from build123d import *

# Parameters (mm, degrees)
F0_R      = 3
F0_R_2    = 0.508
F0_R_3    = 1.375
F3_DEPTH  = 1.2
F4_DEPTH  = 1
F1_W      = 3
F1_H      = 16
F5_DEPTH  = 1
F1_W_2    = 8
F1_H_2    = 5.5
F6_DEPTH  = 2.5
F1_W_3    = 11
F1_H_3    = 7.5
F7_DEPTH  = 3
F8_DEPTH  = 1.2
F1_W_4    = 1.2
F1_H_4    = 8.5
F9_DEPTH  = 1
F2_W      = 12
F2_H      = 12
F2_W_2    = 2.032
F2_H_2    = 1.27
F2_W_3    = 1.27
F2_H_3    = 2.032
F2_W_4    = 2
F2_H_4    = 3
F2_W_5    = 5
F2_W_6    = 3
F2_H_5    = 2.5
F2_W_7    = 2.5
F2_H_6    = 2
F2_W_8    = 1.524
F2_H_7    = 3.048
F10_DEPTH = 1


with BuildPart() as f3:
    # F0 (on Top) → F3 (new body)
    with BuildSketch(Plane.XY):
        with BuildLine():
            ThreePointArc((32.5, 12), (31.62132, 14.12132), (29.5, 15))
            Line((29.5, 15), (-29.5, 15))
            ThreePointArc((-29.5, 15), (-31.62132, 14.12132), (-32.5, 12))
            Line((-32.5, 12), (-32.5, -12))
            ThreePointArc((-32.5, -12), (-31.62132, -14.12132), (-29.5, -15))
            Line((-29.5, -15), (29.5, -15))
            ThreePointArc((29.5, -15), (31.62132, -14.12132), (32.5, -12))
            Line((32.5, -12), (32.5, 12))
        make_face()
        with Locations((-29, -11.5)):
            Circle(F0_R, mode=Mode.SUBTRACT)
        with Locations((29, -11.5)):
            Circle(F0_R, mode=Mode.SUBTRACT)
        with Locations((-24.13, 10.23)):
            Circle(F0_R_2, mode=Mode.SUBTRACT)
        with Locations((-21.59, 10.23)):
            Circle(F0_R_2, mode=Mode.SUBTRACT)
        with Locations((-19.05, 10.23)):
            Circle(F0_R_2, mode=Mode.SUBTRACT)
        with Locations((-16.51, 10.23)):
            Circle(F0_R_2, mode=Mode.SUBTRACT)
        with Locations((-29, 11.5)):
            Circle(F0_R, mode=Mode.SUBTRACT)
        with Locations((-24.13, 12.77)):
            Circle(F0_R_2, mode=Mode.SUBTRACT)
        with Locations((-21.59, 12.77)):
            Circle(F0_R_2, mode=Mode.SUBTRACT)
        with Locations((-19.05, 12.77)):
            Circle(F0_R_2, mode=Mode.SUBTRACT)
        with Locations((-16.51, 12.77)):
            Circle(F0_R_2, mode=Mode.SUBTRACT)
        with Locations((-13.97, 10.23)):
            Circle(F0_R_2, mode=Mode.SUBTRACT)
        with Locations((-11.43, 10.23)):
            Circle(F0_R_2, mode=Mode.SUBTRACT)
        with Locations((-8.89, 10.23)):
            Circle(F0_R_2, mode=Mode.SUBTRACT)
        with Locations((-6.35, 10.23)):
            Circle(F0_R_2, mode=Mode.SUBTRACT)
        with Locations((-3.81, 10.23)):
            Circle(F0_R_2, mode=Mode.SUBTRACT)
        with Locations((-1.27, 10.23)):
            Circle(F0_R_2, mode=Mode.SUBTRACT)
        with Locations((-13.97, 12.77)):
            Circle(F0_R_2, mode=Mode.SUBTRACT)
        with Locations((-11.43, 12.77)):
            Circle(F0_R_2, mode=Mode.SUBTRACT)
        with Locations((-8.89, 12.77)):
            Circle(F0_R_2, mode=Mode.SUBTRACT)
        with Locations((-6.35, 12.77)):
            Circle(F0_R_2, mode=Mode.SUBTRACT)
        with Locations((-3.81, 12.77)):
            Circle(F0_R_2, mode=Mode.SUBTRACT)
        with Locations((-1.27, 12.77)):
            Circle(F0_R_2, mode=Mode.SUBTRACT)
        with Locations((21.59, 5.15)):
            Circle(F0_R_2, mode=Mode.SUBTRACT)
        with Locations((24.13, 5.15)):
            Circle(F0_R_2, mode=Mode.SUBTRACT)
        with Locations((1.27, 10.23)):
            Circle(F0_R_2, mode=Mode.SUBTRACT)
        with Locations((3.81, 10.23)):
            Circle(F0_R_2, mode=Mode.SUBTRACT)
        with Locations((6.35, 10.23)):
            Circle(F0_R_2, mode=Mode.SUBTRACT)
        with Locations((8.89, 10.23)):
            Circle(F0_R_2, mode=Mode.SUBTRACT)
        with Locations((11.43, 10.23)):
            Circle(F0_R_2, mode=Mode.SUBTRACT)
        with Locations((13.97, 10.23)):
            Circle(F0_R_2, mode=Mode.SUBTRACT)
        with Locations((1.27, 12.77)):
            Circle(F0_R_2, mode=Mode.SUBTRACT)
        with Locations((3.81, 12.77)):
            Circle(F0_R_2, mode=Mode.SUBTRACT)
        with Locations((6.35, 12.77)):
            Circle(F0_R_2, mode=Mode.SUBTRACT)
        with Locations((8.89, 12.77)):
            Circle(F0_R_2, mode=Mode.SUBTRACT)
        with Locations((11.43, 12.77)):
            Circle(F0_R_2, mode=Mode.SUBTRACT)
        with Locations((13.97, 12.77)):
            Circle(F0_R_2, mode=Mode.SUBTRACT)
        with Locations((21.59, 7.69)):
            Circle(F0_R_2, mode=Mode.SUBTRACT)
        with Locations((24.13, 7.69)):
            Circle(F0_R_2, mode=Mode.SUBTRACT)
        with Locations((16.51, 10.23)):
            Circle(F0_R_2, mode=Mode.SUBTRACT)
        with Locations((19.05, 10.23)):
            Circle(F0_R_2, mode=Mode.SUBTRACT)
        with Locations((21.59, 10.23)):
            Circle(F0_R_2, mode=Mode.SUBTRACT)
        with Locations((24.13, 10.23)):
            Circle(F0_R_2, mode=Mode.SUBTRACT)
        with Locations((16.51, 12.77)):
            Circle(F0_R_2, mode=Mode.SUBTRACT)
        with Locations((19.05, 12.77)):
            Circle(F0_R_2, mode=Mode.SUBTRACT)
        with Locations((21.59, 12.77)):
            Circle(F0_R_2, mode=Mode.SUBTRACT)
        with Locations((24.13, 12.77)):
            Circle(F0_R_2, mode=Mode.SUBTRACT)
        with Locations((29, 11.5)):
            Circle(F0_R, mode=Mode.SUBTRACT)
        with Locations((-29, -11.5)):
            Circle(F0_R)
        with Locations((-29, -11.5)):
            Circle(F0_R_3, mode=Mode.SUBTRACT)
        with Locations((-29, 11.5)):
            Circle(F0_R)
        with Locations((-29, 11.5)):
            Circle(F0_R_3, mode=Mode.SUBTRACT)
        with Locations((29, 11.5)):
            Circle(F0_R)
        with Locations((29, 11.5)):
            Circle(F0_R_3, mode=Mode.SUBTRACT)
        with Locations((29, -11.5)):
            Circle(F0_R)
        with Locations((29, -11.5)):
            Circle(F0_R_3, mode=Mode.SUBTRACT)
    extrude(amount=-F3_DEPTH)

    # F1 (on Top) → F4 (join)
    with BuildSketch(Plane.XY):
        Polygon((32, -8.5), (33.5, -8.5), (33.5, 8.5), (32, 8.5), (32, 8), (32, -8), align=None)
    extrude(amount=F4_DEPTH)

    # F1 (on Top) → F5 (join)
    with BuildSketch(Plane.XY):
        with Locations((30.5, 0)):
            Rectangle(F1_W, F1_H)
    extrude(amount=F5_DEPTH)

    # F1 (on Top) → F6 (join)
    with BuildSketch(Plane.XY):
        with Locations((21.5, -13.45)):
            Rectangle(F1_W_2, F1_H_2)
        with Locations((8.9, -13.45)):
            Rectangle(F1_W_2, F1_H_2)
    extrude(amount=F6_DEPTH)

    # F1 (on Top) → F7 (join)
    with BuildSketch(Plane.XY):
        with Locations((-20.1, -11.75)):
            Rectangle(F1_W_3, F1_H_3)
    extrude(amount=F7_DEPTH)

    # F1 (on Top) → F8 (join)
    with BuildSketch(Plane.XY):
        Polygon((-19.5, -4.1), (-19.5, 7.9), (-31, 7.9), (-31, 7.4), (-31, 6.9), (-29.8, 6.9), (-29.8, -1.6), (-31, -1.6), (-31, -3.6), (-31, -4.1), align=None)
    extrude(amount=F8_DEPTH)

    # F1 (on Top) → F9 (join)
    with BuildSketch(Plane.XY):
        with Locations((-30.4, 2.65)):
            Rectangle(F1_W_4, F1_H_4)
        with BuildLine():
            Line((-31, 6.9), (-31, 7.4))
            Line((-31, 7.4), (-34, 7.4))
            ThreePointArc((-34, 7.4), (-34.353553, 7.253553), (-34.5, 6.9))
            Line((-34.5, 6.9), (-34.5, -3.1))
            ThreePointArc((-34.5, -3.1), (-34.353553, -3.453553), (-34, -3.6))
            Line((-34, -3.6), (-31, -3.6))
            Line((-31, -3.6), (-31, -1.6))
            Line((-31, -1.6), (-31, 6.9))
        make_face()
    extrude(amount=F9_DEPTH)

    # F2 (on Top) → F10 (join)
    with BuildSketch(Plane.XY):
        with Locations((-6.5, -2)):
            Rectangle(F2_W, F2_H)
        with Locations((-4.516, 7.905)):
            Rectangle(F2_W_2, F2_H_2)
        with Locations((-4.516, 5.635)):
            Rectangle(F2_W_2, F2_H_2)
        with Locations((14.484, -11.865)):
            Rectangle(F2_W_2, F2_H_2)
        with Locations((18.135, -2.984)):
            Rectangle(F2_W_3, F2_H_3)
        with Locations((19.885, -2.984)):
            Rectangle(F2_W_3, F2_H_3)
        with Locations((25.115, -2.5)):
            Rectangle(F2_W_3, F2_H_3)
        with Locations((26.865, -2.5)):
            Rectangle(F2_W_3, F2_H_3)
        with Locations((-14.5, -4.5)):
            Rectangle(F2_W_4, F2_H_4)
        with Locations((11, -1.5)):
            Rectangle(F2_W_5, F2_H_4)
        with Locations((22.5, -2.5)):
            Rectangle(F2_W_6, F2_H_4)
        with Locations((1.5, 6.75)):
            Rectangle(F2_W_4, F2_H_5)
        with Locations((19.75, -6.5)):
            Rectangle(F2_W_7, F2_H_6)
        with Locations((23.238, -7.524)):
            Rectangle(F2_W_8, F2_H_7)
        Polygon((24.2, 4), (23.5, 3.3), (23.5, 1.2), (24.2, 0.5), (26.3, 0.5), (27, 1.2), (27, 3.3), (26.3, 4), align=None)
    extrude(amount=F10_DEPTH)


solid = f3.part
Geometry: final body of the model. Coordinates: model frame, mm. A direction names the side the tool comes from. Give positions to 0.01 mm unless a question says otherwise; leave off trailing zeros. Loops run counter-clockwise (first coordinate to the right, second up) from the corner with the lowest first, then second, coordinate; pieces in that order, holes last. Notation, with made-up numbers: M 65.5,12.5 L 109.5,12.5 A24 cw 109.5,43.5 Z; hole C -30.5,27.25 d7. An arc over 180 degrees is marked long. Put each result on its own line as item: value. Start each with the question number.
1) Contact query for flat-ended pins moving along their axis: pin 1 (6 mm diameter, centred on x = 10, y = -14.5, fed in from +Z); pin 2 (0.9 mm diameter, centred on x = -19.05, y = 12.77, fed in from -Z); pin 3 (1 mm diameter, centred on x = -33.5, y = 4.5, fed in from -Z); pin 4 (1 mm diameter, centred on x = 18.5, y = -3, fed in from +Z). Output: stop coordinate, or through.
2) Pull-direction query (X, two-part tool) for faces 5 (the flat face through (7, 0, 0)), 6 (the flat face through (-25.6, -12, 1)), 7 (the flat face through (11, -1, 1)); classes: pulls with the +X half, pulls with the -X half, needs draft (parallel to the pull), parting line crosses it, or undercut.
3) Access query for faces 1 (the flat face through (18, -3, 1)), 2 (the flat face through (14, -12, 1)), 3 (the flat face through (21, -13, 2.5)), 4 (the flat face through (0, -15, -1)). Directions: +Z, -Z, +X, -X, +Y, -Y. A direction counts if a zero-diameter tool reaches every point of the face in a straight line with its end or side. Return the directions, or none.
4) Cut plane B-B (x = 10). Output: boundary loops of the cut face in (y, z).
5) Ray query, line 1 along Y through (x, z) = (6.35, -0.7); line 2 along Y through (x, z) = (29, -0.75) (3 decimals); line 3 along Y through (x, z) = (9.5, 0.4). Return the intervals inside material, ascending.
6) Cut plane A-A (x = -7.5). Output: boundary loops of the cut face in (y, z).
Verdict:
1. pin 1: z = 2.5
1. pin 2: through
1. pin 3: z = 0
1. pin 4: z = 1
2. face 5: undercut
2. face 6: pulls with the -X half
2. face 7: needs draft
3. face 1: +Z, +X, +Y
3. face 2: +Z, +Y, -Y
3. face 3: +Z, +X, +Y, -Y
3. face 4: -Z, +X, -X, -Y
4. outline: M -16.2,0 L -15,0 L -15,-1.2 L 15,-1.2 L 15,0 L 0,0 L 0,1 L -3,1 L -3,0 L -10.7,0 L -10.7,2.5 L -16.2,2.5 Z
5. line 1: -15 to 9.72, 10.74 to 12.26, 13.28 to 15
5. line 2: -15 to -12.875, -10.125 to 10.125, 12.875 to 15
5. line 3: -16.2 to -10.7, -3 to 0
6. outline: M -15,-1.2 L 15,-1.2 L 15,0 L 4,0 L 4,1 L -8,1 L -8,0 L -15,0 Z
